from build123d import *

# Parameters (mm, degrees)
F0_W     = 7.62
F0_H     = 7.62
F1_DEPTH = 2.54
F2_R     = 2.54
F2_R_2   = 1.27
F3_DEPTH = 22.86
F4_DEPTH = 22.86
F5_DEPTH = 45.72
F6_R     = 0.254
F7_DEPTH = 2.54


# Not quite as in the source:
# - a feature names something its author has since deleted; it is built from what else it names


with BuildPart() as f1:
    # F0 (on Top) → F1 (new body)
    with BuildSketch(Plane.XY):
        with Locations((-38.7955456972, -21.8359371471)):
            Rectangle(F0_W, F0_H)
    extrude(amount=F1_DEPTH)

    # F2 (on face) → F3 (join)
    with BuildSketch(Plane(origin=(0, 0, 0), x_dir=(1, 0, 0), z_dir=(0, 0, -1))):
        with Locations((-38.854431361, 21.8882076442)):
            Circle(F2_R)
        with Locations((-38.854431361, 21.8882076442)):
            Circle(F2_R_2, mode=Mode.SUBTRACT)
    extrude(amount=F3_DEPTH)

    # F4 (add): a face of the model
    f4_faces = [f1.faces().sort_by_distance(p)[0] for p in [
        (-38.854431361, -21.8882076442, 0),
    ]]
    extrude(f4_faces, amount=F4_DEPTH)

    # F2 (on face) → F5 (join)
    with BuildSketch(Plane(origin=(0, 0, 0), x_dir=(1, 0, 0), z_dir=(0, 0, -1))):
        with Locations((-38.854431361, 21.8882076442)):
            Circle(F2_R_2)
    extrude(amount=F5_DEPTH)

    # F6 (on face) → F7 (cut)
    with BuildSketch(Plane(origin=(0, 0, -45.72), x_dir=(1, 0, 0), z_dir=(0, 0, -1))):
        with Locations((-38.854431361, 21.8882076442)):
            Circle(F6_R)
    extrude(amount=-F7_DEPTH, mode=Mode.SUBTRACT)


solid = f1.part
The listing builds one solid part. Answer for the finished solid, in the listing's coordinates (mm). A direction names the side the tool comes from. Coordinates: 2 decimals unless noted, no trailing zeros. Loops run counter-clockwise (first coordinate to the right, second up) from the corner with the lowest first, then second, coordinate; pieces in that order, holes last. Notation, with made-up numbers: (2, 63) -> (16, 63) arc R23 ccw to (16, 80) -> close; hole circle Ø11 at (65, -34.75). An arc over 180 degrees is marked (long way). Write item = value, one per line. Start each with the question number.
1) Given pin 1 Ø1.5 at (x, z) = (-36, -14) entering from -Y; pin 2 Ø3 at (y, z) = (-19.5, -36) entering from +X; pin 3 Ø1 at (x, z) = (-41, -19) entering from +Y, each flat-ended and moving along its own axis, determine where each tip first touches the part or whether it passes through.
2) Straight lines are drawn through the part: line 1 (Z direction, x = -40, y = -23.75); line 2 (Z direction, x = -36.5, y = -24.75); line 3 (X direction, y = -21, z = -35). For each, find the intervals that lie inside material, in ascending order. Write a range as from..to.
3) A cutting plane is placed at B-B (z = -10.5). Give the vertices of the cut face in (x, y).
4) A tool of negligible diameter and unlimited length cuts with its end or side. For faces 1 (the face through (-39.185, -24.407, -11.27)), 2 (the face through (-34.986, -22, 1)), from which of +Z, -Z, +X, -X, +Y, -Y can it reach the whole face along a straight path? Write none if from no direction.
5) A cutting plane is placed at D-D (z = -40). Give the vertices of the cut face in (x, y), then the cut area to 3 significant figures.
6) A cutting plane is placed at A-A (y = -19.75). Give the vertices of the cut face in (x, z).
7) A cutting plane is placed at C-C (y = -24). Give the vertices of the cut face in (x, z), then the cut area to 3 significant figures.
Responses:
q1.pin_1 = -23.31
q1.pin_2 = -37.95
q1.pin_3 = -19.95
q2.line_1 = -22.86..2.54
q2.line_2 = 0..2.54
q2.line_3 = -39.76..-37.95
q3.outline = circle Ø5.08 at (-38.85, -21.89)
q4.face_1 = -Z
q4.face_2 = +Z, -Z, +X, +Y, -Y
q5.outline = circle Ø2.54 at (-38.85, -21.89)
q5.area = 5.07 mm²
q6.outline = (-42.61, 0) -> (-40.23, 0) -> (-40.23, -22.86) -> (-37.48, -22.86) -> (-37.48, 0) -> (-34.99, 0) -> (-34.99, 2.54) -> (-42.61, 2.54) -> close
q7.outline = (-42.61, 0) -> (-40.27, 0) -> (-40.27, -22.86) -> (-37.44, -22.86) -> (-37.44, 0) -> (-34.99, 0) -> (-34.99, 2.54) -> (-42.61, 2.54) -> close
q7.area = 83.9 mm²
